Design review of the part built by this model. Coordinates are the model's own, in mm. Face numbers are marked on the shaded views. A direction names the side the tool comes from. Coordinates: 2 decimals unless noted, no trailing zeros. Order: outer loops, then holes, each group sorted by start corner. A loop starts at its lowest first (then second) coordinate and runs counter-clockwise, first axis right, second up. Notation, with made-up numbers: (45.25, -27) - (87.25, -27) arc R15 cw to (87.25, -19) - close; hole circle Ø1 at (-25.75, 26.25). An arc over 180 degrees is marked (long way). Write item = value, one per line. Start each with the question number.
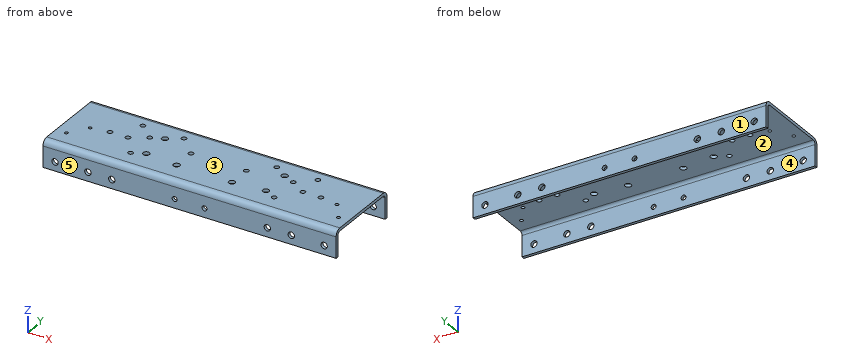
```python
from build123d import *

# Parameters (mm, degrees)
EXTRUDE1_DEPTH           = 311.15
SKETCH2_R                = 5.207
SKETCH2_R_2              = 3.556
SKETCH2_R_3              = 6.731
CUT_WEB_HOLES_DEPTH      = 328.972466987
SKETCH3_R                = 6.731
SKETCH3_R_2              = 5.207
CUT_FLG_HOLES_DEPTH      = 328.972466987
CUT_FLG_HOLES_DEPTH_BACK = 328.972466987


with BuildPart() as part:
    # Sketch1 → Extrude1 (new, symmetric)
    with BuildSketch(Plane(origin=(0, 0, 0), x_dir=(0, 0, -1), z_dir=(1, 0, 0))):
        with BuildLine():
            Line((57.15, 86.51875), (12.7, 86.51875))
            ThreePointArc((12.7, 86.51875), (3.719743879, 82.799006121), (0, 73.81875))
            Line((0, 73.81875), (0, -73.81875))
            ThreePointArc((0, -73.81875), (3.719743879, -82.799006121), (12.7, -86.51875))
            Line((12.7, -86.51875), (57.15, -86.51875))
            Line((57.15, -86.51875), (57.15, -80.16875))
            Line((57.15, -80.16875), (12.7, -80.16875))
            ThreePointArc((12.7, -80.16875), (8.209871939, -78.308878061), (6.35, -73.81875))
            Line((6.35, -73.81875), (6.35, 73.81875))
            ThreePointArc((6.35, 73.81875), (8.209871939, 78.308878061), (12.7, 80.16875))
            Line((12.7, 80.16875), (57.15, 80.16875))
            Line((57.15, 80.16875), (57.15, 86.51875))
        make_face()
    extrude(amount=EXTRUDE1_DEPTH, both=True)

    # Sketch2 → Cut-Web Holes (cut, through all)
    with BuildSketch(Plane.XY):
        with Locations(Location((-152.4, 22.225, 0), (0, 0, 270))):
            Circle(SKETCH2_R)
        with Locations(Location((-185.7375, 52.3875, 0), (0, 0, 270))):
            Circle(SKETCH2_R)
        with Locations(Location((-223.8375, 1.5875, 0), (0, 0, 270))):
            Circle(SKETCH2_R)
        with Locations(Location((-261.9375, -4.7625, 0), (0, 0, 270))):
            Circle(SKETCH2_R_2)
        with Locations(Location((-288.925, -42.8625, 0), (0, 0, 270))):
            Circle(SKETCH2_R_2)
        with Locations(Location((-152.4, -42.8625, 0), (0, 0, 270))):
            Circle(SKETCH2_R)
        with Locations(Location((-127, -30.1625, 0), (0, 0, 270))):
            Circle(SKETCH2_R_3)
        with Locations(Location((-127, 33.3375, 0), (0, 0, 270))):
            Circle(SKETCH2_R_3)
        with Locations(Location((-98.425, 52.3875, 0), (0, 0, 270))):
            Circle(SKETCH2_R)
        with Locations(Location((-58.7375, 12.7, 0), (0, 0, 270))):
            Circle(SKETCH2_R)
        with Locations(Location((-58.7375, -36.5125, 0), (0, 0, 270))):
            Circle(SKETCH2_R_3)
        with Locations(Location((-185.7375, 1.5875, 0), (0, 0, 270))):
            Circle(SKETCH2_R)
        with Locations((98.425, 52.3875)):
            Circle(SKETCH2_R)
        with Locations((127, 33.3375)):
            Circle(SKETCH2_R_3)
        with Locations((152.4, 22.225)):
            Circle(SKETCH2_R)
        with Locations((185.7375, 52.3875)):
            Circle(SKETCH2_R)
        with Locations((223.8375, 1.5875)):
            Circle(SKETCH2_R)
        with Locations((185.7375, 1.5875)):
            Circle(SKETCH2_R)
        with Locations((261.9375, -4.7625)):
            Circle(SKETCH2_R_2)
        with Locations((288.925, -42.8625)):
            Circle(SKETCH2_R_2)
        with Locations((152.4, -42.8625)):
            Circle(SKETCH2_R)
        with Locations((127, -30.1625)):
            Circle(SKETCH2_R_3)
        with Locations((58.7375, 12.7)):
            Circle(SKETCH2_R)
        with Locations((58.7375, -36.5125)):
            Circle(SKETCH2_R_3)
    extrude(amount=-CUT_WEB_HOLES_DEPTH, mode=Mode.SUBTRACT)

    # Sketch3 → Cut-Flg Holes (cut, two sides)
    with BuildSketch(Plane(origin=(0, 0, 0), x_dir=(1, 0, 0), z_dir=(0, 1, 0))) as cut_flg_holes_sk:
        with Locations(Location((-285.75, 38.1, 0), (0, 0, 270))):
            Circle(SKETCH3_R)
        with Locations(Location((-215.9, 38.1, 0), (0, 0, 270))):
            Circle(SKETCH3_R)
        with Locations(Location((285.75, 38.1, 0), (0, 0, 90))):
            Circle(SKETCH3_R)
        with Locations(Location((215.9, 38.1, 0), (0, 0, 90))):
            Circle(SKETCH3_R)
        with Locations(Location((165.1, 38.1, 0), (0, 0, 270))):
            Circle(SKETCH3_R)
        with Locations(Location((31.75, 38.1, 0), (0, 0, 270))):
            Circle(SKETCH3_R_2)
        with Locations(Location((-31.75, 38.1, 0), (0, 0, 270))):
            Circle(SKETCH3_R_2)
        with Locations(Location((-165.1, 38.1, 0), (0, 0, 270))):
            Circle(SKETCH3_R)
    extrude(amount=CUT_FLG_HOLES_DEPTH, mode=Mode.SUBTRACT)
    extrude(cut_flg_holes_sk.sketch, amount=-CUT_FLG_HOLES_DEPTH_BACK, mode=Mode.SUBTRACT)


solid = part.part
```
Item 1: Add section A-A on x = 31.75. Give the boundary of the cut face in (y, z), plus the area to 3 significant figures.
Item 2: For the marked faces 1 and 2, list the 3-axis set-ups (+Z, -Z, +X, -X, +Y, -Y) from which the entire face can be reached by the end or side of a thin tool; tool diameter is ignored.
Item 3: Add section C-C on x = 127. Give the boundary of the cut face in (y, z).
Item 4: Add section B-B on z = -51. Give the boundary of the cut face in (x, y), plus the area to 3 significant figures.
Item 5: For P1, Ø17.5, axis at x = 165.1, z = -38.1, coming from the +Y side; P2, Ø11, axis at x = -165.1, z = -38.1, coming from the -Y side; P3, Ø1.5, axis at x = -147.5, y = 6, coming from the -Z side, all flat-tipped, find the tip position at first contact; note any pin that passes through.
Item 6: For line 1 (Y direction, x = -174.5, z = -19); line 2 (Y direction, x = 153.5, z = -3.5); line 3 (Z direction, x = 29.5, y = 61.5), list the stretches that pass through material, from the lowest coordinate up.
Item 7: Mouldability with a two-part tool opening along Y and no side actions: class the marked faces 3, 4 and 5 as +Y half, -Y half, draft (parallel to the pull), parting line (faces both ways), or undercut.
Worked out:
q1.outline = (-86.52, -57.15) - (-80.17, -57.15) - (-80.17, -43.31) - (-86.52, -43.31) - close; (-86.52, -32.89) - (-80.17, -32.89) - (-80.17, -12.7) arc R6.35 cw to (-73.82, -6.35) - (73.82, -6.35) arc R6.35 cw to (80.17, -12.7) - (80.17, -32.89) - (86.52, -32.89) - (86.52, -12.7) arc R12.7 ccw to (73.82, 0) - (-73.82, 0) arc R12.7 ccw to (-86.52, -12.7) - close; (80.17, -57.15) - (86.52, -57.15) - (86.52, -43.31) - (80.17, -43.31) - close
q1.area = 1,560 mm2
q2.face_1 = +Z, -Z, +X, -X, +Y
q2.face_2 = -Z, +X, -X
q3.outline = (-86.52, -57.15) - (-80.17, -57.15) - (-80.17, -12.7) arc R6.35 cw to (-73.82, -6.35) - (-36.89, -6.35) - (-36.89, 0) - (-73.82, 0) arc R12.7 ccw to (-86.52, -12.7) - close; (-23.43, -6.35) - (26.61, -6.35) - (26.61, 0) - (-23.43, 0) - close; (40.07, -6.35) - (73.82, -6.35) arc R6.35 cw to (80.17, -12.7) - (80.17, -57.15) - (86.52, -57.15) - (86.52, -12.7) arc R12.7 ccw to (73.82, 0) - (40.07, 0) - close
q4.outline = (-311.15, -86.52) - (311.15, -86.52) - (311.15, -80.17) - (-311.15, -80.17) - close; (-311.15, 80.17) - (311.15, 80.17) - (311.15, 86.52) - (-311.15, 86.52) - close
q4.area = 7,900 mm2
q5.P1 = 86.52
q5.P2 = through
q5.P3 = -6.35
q6.line_1 = -86.52 to -80.17, 80.17 to 86.52
q6.line_2 = -82.57 to -47.95, -37.77 to 17.14, 27.31 to 82.57
q6.line_3 = -6.35 to 0
q7.face_3 = draft
q7.face_4 = undercut
q7.face_5 = -Y half
